```python
from build123d import *

# Parameters (mm, degrees)
SKETCH_1_W             = 300
SKETCH_1_H             = 205
SM_BASE_FLANGE_1_DEPTH = 10
CHAMFER_1_SIZE         = 8
CHAMFER_1_SIZE2        = 5.601660306
CHAMFER_2_SIZE         = 8
CHAMFER_2_SIZE2        = 5.601660306


# Sheet-metal steps are written as plain solids
with BuildPart() as part:
    # Sketch 1 → 基体-法兰1 (new body)
    with BuildSketch(Plane.XY):
        Rectangle(SKETCH_1_W, SKETCH_1_H)
    extrude(amount=-SM_BASE_FLANGE_1_DEPTH)

    # 倒角1
    chamfer_1_edges = [part.edges().sort_by_distance(p)[0] for p in [
        (0, 102.5, -10),
    ]]
    chamfer_1_side = [part.faces().sort_by_distance(p)[0] for p in [
        (0, 102.5, -5),
    ]]
    chamfer(chamfer_1_edges, length=CHAMFER_1_SIZE, length2=CHAMFER_1_SIZE2, reference=chamfer_1_side[0])

    # 倒角2
    chamfer_2_edges = [part.edges().sort_by_distance(p)[0] for p in [
        (0, -102.5, -10),
    ]]
    chamfer_2_side = [part.faces().sort_by_distance(p)[0] for p in [
        (0, -102.5, -5),
    ]]
    chamfer(chamfer_2_edges, length=CHAMFER_2_SIZE, length2=CHAMFER_2_SIZE2, reference=chamfer_2_side[0])


solid = part.part
```
Work out the finished part from the listing and answer in its coordinate system (mm). Give positions to 0.01 mm unless a question says otherwise; leave off trailing zeros. Order: outer loops, then holes, each group sorted by start corner. A loop starts at its lowest first (then second) coordinate and runs counter-clockwise, first axis right, second up. Notation, with made-up numbers: (77.5, 89) - (128.5, 89) arc R28 ccw to (128.5, 117) - close; hole circle Ø2 at (72.5, 77.5). An arc over 180 degrees is marked (long way). One line per item, written item: value. Start each with the question number.
1. This flat-tipped pin is pushed along its axis until it touches: pin 1 Ø6 at (x, z) = (57, -3.5) entering from -Y. Where does it stop, or does it pass through?
2. Section B-B, the plane z = -4.75 is taken. Write down the section's boundary in (x, y).
3. Consider line 1 (Y direction, x = 34, z = -4.25); line 2 (Y direction, x = -104.5, z = -8.75). Determine where each line is inside the solid, lowest interval first.
4. Section A-A, the plane x = 103.5 is taken. Write down the section's boundary in (y, z).
Filled sheet:
1. pin 1: y = -102.5
2. outline: (-150, -100.57) - (150, -100.57) - (150, 100.57) - (-150, 100.57) - close
3. line 1: -100.92 to 100.92
3. line 2: -97.77 to 97.77
4. outline: (-102.5, -2) - (-96.9, -10) - (96.9, -10) - (102.5, -2) - (102.5, 0) - (-102.5, 0) - close
